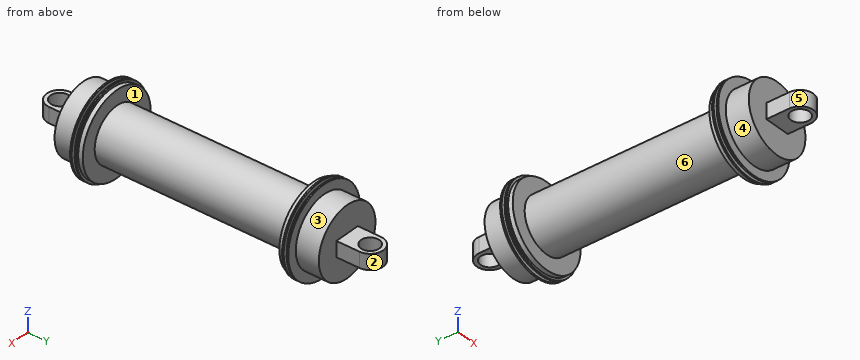
from build123d import *

# Parameters (mm, degrees)
SKETCH1_R           = 17.5
BOSS_EXTRUDE1_DEPTH = 142
SHELL1_T            = -2
SKETCH2_R           = 22.5
BOSS_EXTRUDE2_DEPTH = 15
SKETCH3_R           = 6
BOSS_EXTRUDE3_DEPTH = 5
SKETCH4_R           = 28.5
BOSS_EXTRUDE4_DEPTH = 1
SKETCH5_R           = 26
BOSS_EXTRUDE5_DEPTH = 2
SKETCH6_R           = 28.5
BOSS_EXTRUDE6_DEPTH = 1
SKETCH7_R           = 27
BOSS_EXTRUDE7_DEPTH = 3


with BuildPart() as part:
    # Sketch1 → Boss-Extrude1 (new body)
    with BuildSketch(Plane(origin=(0, 0, 0), x_dir=(1, 0, 0), z_dir=(0, 1, 0))):
        with Locations(Location((0, 0, 0), (0, 0, 270))):
            Circle(SKETCH1_R)
    extrude(amount=BOSS_EXTRUDE1_DEPTH)

    # Shell1
    shell1_openings = [part.faces().sort_by_distance(p)[0] for p in [
        (0, 142, 0),
        (0, 0, 0),
    ]]
    offset(amount=SHELL1_T, openings=shell1_openings, kind=Kind.INTERSECTION)

    # Sketch2 → Boss-Extrude2 (add)
    with BuildSketch(Plane.XZ):
        with Locations(Location((0, 0, 0), (0, 0, 270))):
            Circle(SKETCH2_R)
    boss_extrude2 = extrude(amount=BOSS_EXTRUDE2_DEPTH)

    # Sketch3 → Boss-Extrude3 (add, symmetric)
    with BuildSketch(Plane.XY):
        with BuildLine():
            Line((-8.5, -15), (-8.5, -30))
            ThreePointArc((-8.5, -30), (0, -38.5), (8.5, -30))
            Line((8.5, -30), (8.5, -15))
            Line((8.5, -15), (-8.5, -15))
        make_face()
        with Locations((0, -30)):
            Circle(SKETCH3_R, mode=Mode.SUBTRACT)
    boss_extrude3 = extrude(amount=BOSS_EXTRUDE3_DEPTH, both=True)

    # Mirror1: Boss-Extrude2, Boss-Extrude3 across plane
    add(boss_extrude2.mirror(Plane.ZX.offset(71)))
    add(boss_extrude3.mirror(Plane.ZX.offset(71)))

    # Sketch4 → Boss-Extrude4 (add)
    with BuildSketch(Plane.XZ.offset(-142)):
        with Locations(Location((0, 0, 0), (0, 0, 270))):
            Circle(SKETCH4_R)
    boss_extrude4 = extrude(amount=BOSS_EXTRUDE4_DEPTH)

    # Sketch5 → Boss-Extrude5 (add)
    with BuildSketch(Plane.XZ.offset(-141)):
        with Locations(Location((0, 0, 0), (0, 0, 270))):
            Circle(SKETCH5_R)
    boss_extrude5 = extrude(amount=BOSS_EXTRUDE5_DEPTH)

    # Sketch6 → Boss-Extrude6 (add)
    with BuildSketch(Plane.XZ.offset(-139)):
        with Locations(Location((0, 0, 0), (0, 0, 270))):
            Circle(SKETCH6_R)
    boss_extrude6 = extrude(amount=BOSS_EXTRUDE6_DEPTH)

    # Mirror2: Boss-Extrude4, Boss-Extrude5, Boss-Extrude6 across plane
    add(boss_extrude4.mirror(Plane.ZX.offset(71)))
    add(boss_extrude5.mirror(Plane.ZX.offset(71)))
    add(boss_extrude6.mirror(Plane.ZX.offset(71)))

    # Sketch7 → Boss-Extrude7 (add)
    with BuildSketch(Plane.XZ.offset(-138)):
        with Locations(Location((0, 0, 0), (0, 0, 270))):
            Circle(SKETCH7_R)
    boss_extrude7 = extrude(amount=BOSS_EXTRUDE7_DEPTH)

    # Mirror3: Boss-Extrude7 across plane
    add(boss_extrude7.mirror(Plane.ZX.offset(71)))


solid = part.part
Input: part model. Units: mm. Frame: model coordinates. Face numbers are marked on the shaded views. A direction names the side the tool comes from. Give positions to 0.01 mm unless a question says otherwise; leave off trailing zeros. Write each loop counter-clockwise with the first axis right and the second up, starting at its lowest first coordinate (ties: lowest second). Pieces come first, ordered by that corner, then holes.
Q1. Section D-D, the plane y = -7.5. Output: boundary loops of the cut face in (x, z), plus the area to 3 significant figures.
Q2. Set-up query: the marked faces 4, 5 and 6. Return all of +Z, -Z, +X, -X, +Y, -Y with unobstructed straight access to the full face (end or side cutting, diameter ignored); none if empty.
Q3. Section C-C, the plane y = 107. Output: boundary loops of the cut face in (x, z), plus the area to 3 significant figures.
Q4. Material intervals for probe 1 along Y at (x, z) = (-25, 10); probe 2 along Y at (x, z) = (0, 2.5); probe 3 along X at (y, z) = (104, 0), sorted ascending.
Q5. Pull-direction query (Y, two-part tool) for the marked faces 1, 2 and 3; classes: pulls with the +Y half, pulls with the -Y half, needs draft (parallel to the pull), parting line crosses it, or undercut.
Q6. First-contact query: P1, Ø4, axis at x = -21, y = 15.5, coming from the +Z side; P2, Ø1, axis at x = 1, y = 149.5, coming from the +Z side; P3, Ø4, axis at y = -7.5, z = -13.5, coming from the -X side; P4, Ø15.5, axis at x = 0, y = -30, coming from the -Z side. Flat tips, straight axial feed; report the tip coordinate or a pass-through.
Q7. Section A-A, the plane x = 0. State how many separate pieces and enclosed holes the cut face has, plus the area to 3 significant figures.
Filled in:
1. outline: circle Ø45 at (0, 0)
1. area: 1,590 mm2
2. face 4: -Y
2. face 5: +Z, -Z, -Y
2. face 6: none
3. outline: circle Ø35 at (0, 0); hole circle Ø31 at (0, 0)
3. area: 207 mm2
4. probe 1: y = 0 to 1, 3 to 7, 135 to 139, 141 to 142
4. probe 2: y = -38.5 to -36, -24 to 7, 135 to 166, 178 to 180.5
4. probe 3: x = -17.5 to -15.5, 15.5 to 17.5
5. face 1: undercut
5. face 2: pulls with the +Y half
5. face 3: needs draft
6. P1: passes through
6. P2: stops at z = 22.49
6. P3: stops at x = -19.34
6. P4: stops at z = -5
7. separate pieces: 3
7. enclosed holes: 1
7. area: 2,850 mm2
